```python
from build123d import *

# Parameters (mm, degrees)
F1_DEPTH = 6
F2_R     = 2
F3_DEPTH = 25
F4_R     = 2
F5_DEPTH = 10


with BuildPart() as f1:
    # F0 (on Front) → F1 (new body)
    with BuildSketch(Plane.XZ):
        Polygon((-38.636893, 10.616255), (-45.869478, 10.616255), (-45.869478, -8.383745), (-38.722239, -8.383745), (-40.275154, -2.58819), (-30.615895, 0), (-28.369478, -8.383745), (63.630522, -8.383745), (84.130522, -2.890787), (84.130522, 4.616255), (-7.869478, 4.616255), (-20.869478, 10.616255), (-33.460512, 10.616255), (-32.425236, 6.752551), (-37.254865, 5.458456), align=None)
    extrude(amount=F1_DEPTH)

    # F2 (on Front) + F1_face (on face) → F3 (cut)
    with BuildSketch(Plane.XZ):
        with Locations((76.130522, -1.383745)):
            Circle(F2_R)
    with BuildSketch(Plane(origin=(14.871895, -6, -0.728123), x_dir=(1, 0, 0), z_dir=(0, -1, 0))):
        Polygon((-52.12676, 6.186579), (-53.508788, 11.344377), (-60.741372, 11.344377), (-60.741372, -7.655623), (-53.594134, -7.655623), (-55.147048, -1.860068), (-45.48779, 0.728123), (-43.241372, -7.655623), (48.758628, -7.655623), (69.258628, -2.162664), (69.258628, 5.344377), (-22.741372, 5.344377), (-35.741372, 11.344377), (-48.332407, 11.344377), (-47.297131, 7.480674), align=None)
    extrude(amount=F3_DEPTH, mode=Mode.SUBTRACT)

    # F4 (on face) → F5 (cut)
    with BuildSketch(Plane(origin=(6.358373, 0, -23.729772), x_dir=(0.965926, 0, 0.258819), z_dir=(0.258819, 0, -0.965926))):
        with Locations((68.515654, 3)):
            Circle(F4_R)
    extrude(amount=-F5_DEPTH, mode=Mode.SUBTRACT)


solid = f1.part
```
Geometry: final body of the model. Coordinates: model frame, mm. A direction names the side the tool comes from. Give positions to 0.01 mm unless a question says otherwise; leave off trailing zeros. Loops run counter-clockwise (first coordinate to the right, second up) from the corner with the lowest first, then second, coordinate; pieces in that order, holes last. Notation, with made-up numbers: (-16, 68) -> (39, 68) arc R23 ccw to (39, 85) -> close; hole circle Ø3 at (89.5, 35). An arc over 180 degrees is marked (long way). Use one line per item in the form item = value.
Item 1: Pin query (flat end, axial travel): P1, Ø4.5, axis at x = 76.13, z = -1.38, coming from the +Y side; P2, Ø1.8, axis at x = 24, y = -3.5, coming from the +Z side. Return the tip coordinate at first contact, or that it passes through.
A:
P1 = 0
P2 = 4.62
Item 2: Line query: probe 1 along Z at (x, y) = (16, -4.9); probe 2 along X at (y, z) = (-2.7, -6.25); probe 3 along X at (y, z) = (-0.95, 10). Output: solid intervals per line, ascending.
A:
probe_1 = -8.38 to 4.62
probe_2 = -45.87 to -39.29, -28.94 to 70.56
probe_3 = -45.87 to -38.47, -33.3 to -19.53
Item 3: Section query A-A on y = -1.9. Output: boundary loops of the cut face in (x, z).
A:
outline = (-45.87, -8.38) -> (-38.72, -8.38) -> (-40.28, -2.59) -> (-30.62, 0) -> (-28.37, -8.38) -> (63.63, -8.38) -> (70.93, -6.43) -> (68.34, 3.23) -> (71.56, 4.09) -> (74.15, -5.56) -> (84.13, -2.89) -> (84.13, 4.62) -> (-7.87, 4.62) -> (-20.87, 10.62) -> (-33.46, 10.62) -> (-32.43, 6.75) -> (-37.25, 5.46) -> (-38.64, 10.62) -> (-45.87, 10.62) -> close; hole circle Ø4 at (76.13, -1.38)
Item 4: Draft query along Z for faces 1 (the face through (-39.488, -2.958, -5.527)), 2 (the face through (-29.51, -2.96, -4.13)), 3 (the face through (-14.278, -2.958, 7.574)). Return one class per face: pulls with the +Z half, pulls with the -Z half, needs draft (parallel to the pull), parting line crosses it, or undercut.
A:
face_1 = undercut
face_2 = pulls with the -Z half
face_3 = pulls with the +Z half
Item 5: Section query B-B on x = 4. Output: boundary loops of the cut face in (y, z).
A:
outline = (-6, -8.38) -> (0, -8.38) -> (0, 4.62) -> (-6, 4.62) -> close
Item 6: Access query for faces 4 (the face through (69.924, -3.028, 3.655)), 5 (the face through (-37.936, -2.958, 8.001)), 6 (the face through (-34.806, -2.958, 6.115)). Directions: +Z, -Z, +X, -X, +Y, -Y. A direction counts if a zero-diameter tool reaches every point of the face in a straight line with its end or side. Return the directions, or none.
A:
face_4 = none
face_5 = +Z, +Y, -Y
face_6 = +Y, -Y
